```python
from build123d import *

# Parameters (mm, degrees)
SKETCH1_W                     = 220
SKETCH1_H                     = 350
BOSS_EXTRUDE1_DEPTH           = 5
SKETCH2_W                     = 49.4
SKETCH2_H                     = 69.5
BOSS_EXTRUDE2_DEPTH           = 26
LPATTERN1_COUNT               = 2
LPATTERN1_PITCH               = 50
LPATTERN3_COUNT               = 3
LPATTERN3_PITCH               = 70
LPATTERN3_COPY_1_SKETCH_W     = 49.4
LPATTERN3_COPY_1_SKETCH_H     = 69.5
LPATTERN3_COPY_1_DEPTH        = 26
LPATTERN3_COPY_2_SKETCH_W     = 49.4
LPATTERN3_COPY_2_SKETCH_H     = 69.5
LPATTERN3_COPY_2_DEPTH        = 26
LPATTERN3_COL_COUNT           = 3
LPATTERN3_COL_PITCH           = 70
LPATTERN3_COL_COPY_1_SKETCH_W = 49.4
LPATTERN3_COL_COPY_1_SKETCH_H = 69.5
LPATTERN3_COL_COPY_1_DEPTH    = 26
LPATTERN3_COL_COPY_2_SKETCH_W = 49.4
LPATTERN3_COL_COPY_2_SKETCH_H = 69.5
LPATTERN3_COL_COPY_2_DEPTH    = 26
SKETCH4_W                     = 69.5
SKETCH4_H                     = 49.5
BOSS_EXTRUDE3_DEPTH           = 26
LPATTERN4_COUNT               = 3
LPATTERN4_PITCH               = 50
LPATTERN4_COL_COUNT           = 3
LPATTERN4_COL_PITCH           = 50
LPATTERN5_COUNT               = 2
LPATTERN5_PITCH               = 170
LPATTERN5_COPY_1_SKETCH_W     = 69.5
LPATTERN5_COPY_1_SKETCH_H     = 49.5
LPATTERN5_COPY_1_DEPTH        = 26
LPATTERN5_COPY_2_SKETCH_W     = 69.5
LPATTERN5_COPY_2_SKETCH_H     = 49.5
LPATTERN5_COPY_2_DEPTH        = 26
LPATTERN5_COPY_3_SKETCH_W     = 69.5
LPATTERN5_COPY_3_SKETCH_H     = 49.5
LPATTERN5_COPY_3_DEPTH        = 26
LPATTERN5_COPY_4_SKETCH_W     = 69.5
LPATTERN5_COPY_4_SKETCH_H     = 49.5
LPATTERN5_COPY_4_DEPTH        = 26


with BuildPart() as part:
    # Sketch1 → Boss-Extrude1 (new body)
    with BuildSketch(Plane(origin=(0, 0, 0), x_dir=(1, 0, 0), z_dir=(0, 1, 0))):
        Rectangle(SKETCH1_W, SKETCH1_H)
    extrude(amount=BOSS_EXTRUDE1_DEPTH)

    # Sketch2 → Boss-Extrude2 (add)
    with BuildSketch(Plane(origin=(0, 5, 0), x_dir=(1, 0, 0), z_dir=(0, 1, 0))):
        with Locations((-24.8, 0)):
            Rectangle(SKETCH2_W, SKETCH2_H)
    boss_extrude2 = extrude(amount=BOSS_EXTRUDE2_DEPTH)

    # LPattern1: Boss-Extrude2 ×2
    with Locations(*[(i * LPATTERN1_PITCH, 0, 0) for i in range(1, LPATTERN1_COUNT)]):
        add(boss_extrude2)

    # LPattern3: Boss-Extrude2 ×3
    with Locations(*[(0, 0, -i * LPATTERN3_PITCH) for i in range(1, LPATTERN3_COUNT)]):
        add(boss_extrude2)

    # LPattern3 copy 1 sketch → LPattern3 copy 1 (add)
    with BuildSketch(Plane(origin=(50, 5, -70), x_dir=(1, 0, 0), z_dir=(0, 1, 0))):
        with Locations((-24.8, 0)):
            Rectangle(LPATTERN3_COPY_1_SKETCH_W, LPATTERN3_COPY_1_SKETCH_H)
    extrude(amount=LPATTERN3_COPY_1_DEPTH)

    # LPattern3 copy 2 sketch → LPattern3 copy 2 (add)
    with BuildSketch(Plane(origin=(50, 5, -140), x_dir=(1, 0, 0), z_dir=(0, 1, 0))):
        with Locations((-24.8, 0)):
            Rectangle(LPATTERN3_COPY_2_SKETCH_W, LPATTERN3_COPY_2_SKETCH_H)
    extrude(amount=LPATTERN3_COPY_2_DEPTH)

    # LPattern3 col: Boss-Extrude2 ×3
    with Locations(*[(0, 0, i * LPATTERN3_COL_PITCH) for i in range(1, LPATTERN3_COL_COUNT)]):
        add(boss_extrude2)

    # LPattern3 col copy 1 sketch → LPattern3 col copy 1 (add)
    with BuildSketch(Plane(origin=(50, 5, 70), x_dir=(1, 0, 0), z_dir=(0, 1, 0))):
        with Locations((-24.8, 0)):
            Rectangle(LPATTERN3_COL_COPY_1_SKETCH_W, LPATTERN3_COL_COPY_1_SKETCH_H)
    extrude(amount=LPATTERN3_COL_COPY_1_DEPTH)

    # LPattern3 col copy 2 sketch → LPattern3 col copy 2 (add)
    with BuildSketch(Plane(origin=(50, 5, 140), x_dir=(1, 0, 0), z_dir=(0, 1, 0))):
        with Locations((-24.8, 0)):
            Rectangle(LPATTERN3_COL_COPY_2_SKETCH_W, LPATTERN3_COL_COPY_2_SKETCH_H)
    extrude(amount=LPATTERN3_COL_COPY_2_DEPTH)

    # Sketch4 → Boss-Extrude3 (add)
    with BuildSketch(Plane(origin=(0, 5, 0), x_dir=(1, 0, 0), z_dir=(0, 1, 0))):
        with Locations((-84.35, 0)):
            Rectangle(SKETCH4_W, SKETCH4_H)
    boss_extrude3 = extrude(amount=BOSS_EXTRUDE3_DEPTH)

    # LPattern4: Boss-Extrude3 ×3
    with Locations(*[(0, 0, i * LPATTERN4_PITCH) for i in range(1, LPATTERN4_COUNT)]):
        add(boss_extrude3)

    # LPattern4 col: Boss-Extrude3 ×3
    with Locations(*[(0, 0, -i * LPATTERN4_COL_PITCH) for i in range(1, LPATTERN4_COL_COUNT)]):
        add(boss_extrude3)

    # LPattern5: Boss-Extrude3 ×2
    with Locations(*[(i * LPATTERN5_PITCH, 0, 0) for i in range(1, LPATTERN5_COUNT)]):
        add(boss_extrude3)

    # LPattern5 copy 1 sketch → LPattern5 copy 1 (add)
    with BuildSketch(Plane(origin=(170, 5, 50), x_dir=(1, 0, 0), z_dir=(0, 1, 0))):
        with Locations((-84.35, 0)):
            Rectangle(LPATTERN5_COPY_1_SKETCH_W, LPATTERN5_COPY_1_SKETCH_H)
    extrude(amount=LPATTERN5_COPY_1_DEPTH)

    # LPattern5 copy 2 sketch → LPattern5 copy 2 (add)
    with BuildSketch(Plane(origin=(170, 5, 100), x_dir=(1, 0, 0), z_dir=(0, 1, 0))):
        with Locations((-84.35, 0)):
            Rectangle(LPATTERN5_COPY_2_SKETCH_W, LPATTERN5_COPY_2_SKETCH_H)
    extrude(amount=LPATTERN5_COPY_2_DEPTH)

    # LPattern5 copy 3 sketch → LPattern5 copy 3 (add)
    with BuildSketch(Plane(origin=(170, 5, -50), x_dir=(1, 0, 0), z_dir=(0, 1, 0))):
        with Locations((-84.35, 0)):
            Rectangle(LPATTERN5_COPY_3_SKETCH_W, LPATTERN5_COPY_3_SKETCH_H)
    extrude(amount=LPATTERN5_COPY_3_DEPTH)

    # LPattern5 copy 4 sketch → LPattern5 copy 4 (add)
    with BuildSketch(Plane(origin=(170, 5, -100), x_dir=(1, 0, 0), z_dir=(0, 1, 0))):
        with Locations((-84.35, 0)):
            Rectangle(LPATTERN5_COPY_4_SKETCH_W, LPATTERN5_COPY_4_SKETCH_H)
    extrude(amount=LPATTERN5_COPY_4_DEPTH)


solid = part.part
```
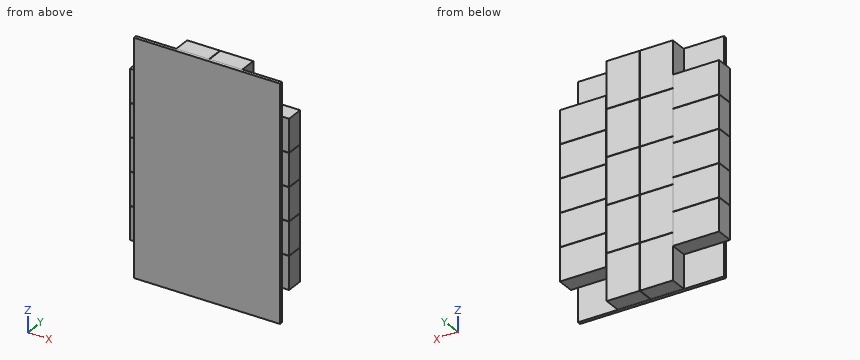
Geometry check sheet. Reference: the model listing, model coordinates, mm. Give positions to 0.01 mm unless a question says otherwise; leave off trailing zeros. Write each loop counter-clockwise with the first axis right and the second up, starting at its lowest first coordinate (ties: lowest second). Pieces come first, ordered by that corner, then holes. Notation, with made-up numbers: (33, 27) -> (56, 27) arc R18 cw to (56, 49) -> close; hole circle Ø7 at (-8.75, 30.5). An arc over 180 degrees is marked (long way). Use one line per item in the form item = value.
Item 1: Sectioned sample at A-A on x = 60. Enter the section's corners in (y, z), plus the area to 4 significant figures.
Results list:
outline = (0, -175) -> (5, -175) -> (5, -124.75) -> (31, -124.75) -> (31, -75.25) -> (5, -75.25) -> (5, -74.75) -> (31, -74.75) -> (31, -25.25) -> (5, -25.25) -> (5, -24.75) -> (31, -24.75) -> (31, 24.75) -> (5, 24.75) -> (5, 25.25) -> (31, 25.25) -> (31, 74.75) -> (5, 74.75) -> (5, 75.25) -> (31, 75.25) -> (31, 124.75) -> (5, 124.75) -> (5, 175) -> (0, 175) -> close
area = 8,185 mm2
Item 2: Sectioned sample at B-B on z = -111. Enter the section's corners in (x, y).
Results list:
outline = (-119.1, 5) -> (-110, 5) -> (-110, 0) -> (110, 0) -> (110, 5) -> (120.4, 5) -> (120.4, 31) -> (50.9, 31) -> (50.9, 5) -> (49.9, 5) -> (49.9, 31) -> (0.5, 31) -> (0.5, 5) -> (-0.1, 5) -> (-0.1, 31) -> (-49.5, 31) -> (-49.5, 5) -> (-49.6, 5) -> (-49.6, 31) -> (-119.1, 31) -> close
Item 3: Depth check by flat-ended pin: pin 1 Ø1.5 at (y, z) = (3.5, 35) entering from -X; pin 2 Ø8 at (x, y) = (94, 23.5) entering from +Z; pin 3 Ø1.5 at (x, y) = (6.5, 14.5) entering from -Z; pin 4 Ø5.5 at (y, z) = (3.5, -60.5) entering from +X. Enter the tip coordinate at first touch or a pass-through.
Results list:
pin_1 = -110
pin_2 = 124.75
pin_3 = -174.75
pin_4 = 120.4
Item 4: Scan lines: line 1 (Z direction, x = 88, y = 9); line 2 (Z direction, x = 38, y = 30.5); line 3 (Y direction, x = 59, z = -126). Record each from-to range of solid material in increasing order.
Results list:
line_1 = -124.75 to -75.25, -74.75 to -25.25, -24.75 to 24.75, 25.25 to 74.75, 75.25 to 124.75
line_2 = -174.75 to -105.25, -104.75 to -35.25, -34.75 to 34.75, 35.25 to 104.75, 105.25 to 174.75
line_3 = 0 to 5
Item 5: Sectioned sample at C-C on y = 8.5. Count the separate pieces of the cut face and the enclosed holes in it, plus the area to 3 significant figures.
Results list:
separate_pieces = 20
enclosed_holes = 0
area = 68,700 mm2
